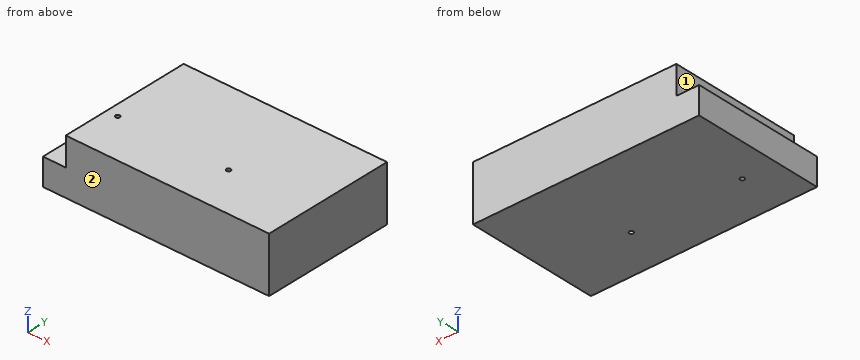
from build123d import *

# Parameters (mm, degrees)
SKETCH_1_W          = 159
SKETCH_1_H          = 93
EXTRUDE_1_DEPTH     = 39
SKETCH_2_R          = 1.5
CUT_EXTRUDE_1_DEPTH = 39
SKETCH_3_W          = 16
SKETCH_3_H          = 93
CUT_EXTRUDE_2_DEPTH = 20


with BuildPart() as part:
    # Эскиз1 → Бобышка-Вытянуть1 (new body)
    with BuildSketch(Plane.XY):
        Rectangle(SKETCH_1_W, SKETCH_1_H)
    extrude(amount=EXTRUDE_1_DEPTH)

    # Эскиз2 → Вырез-Вытянуть1 (cut)
    with BuildSketch(Plane(origin=(0, 0, 0), x_dir=(-1, 0, 0), z_dir=(0, 0, -1))):
        with Locations((-22.5, -14.5)):
            Circle(SKETCH_2_R)
        with Locations((55.5, -14.5)):
            Circle(SKETCH_2_R)
    extrude(amount=-CUT_EXTRUDE_1_DEPTH, mode=Mode.SUBTRACT)

    # Эскиз3 → Вырез-Вытянуть2 (cut)
    with BuildSketch(Plane.XY.offset(39)):
        with Locations((-71.5, 0)):
            Rectangle(SKETCH_3_W, SKETCH_3_H)
    extrude(amount=-CUT_EXTRUDE_2_DEPTH, mode=Mode.SUBTRACT)


solid = part.part
Geometry: final body of the model. Coordinates: model frame, mm. Face numbers are marked on the shaded views. A direction names the side the tool comes from. Give positions to 0.01 mm unless a question says otherwise; leave off trailing zeros. Write each loop counter-clockwise with the first axis right and the second up, starting at its lowest first coordinate (ties: lowest second). Pieces come first, ordered by that corner, then holes. Notation, with made-up numbers: (56.5, 27) -> (67.5, 27) arc R22 cw to (67.5, 35) -> close; hole circle Ø8 at (-15, 83). An arc over 180 degrees is marked (long way). Answer as a JSON object with one key per item and string values.
1. Ray query, probe 1 along X at (y, z) = (-14, 10); probe 2 along Y at (x, z) = (22.5, 31); probe 3 along X at (y, z) = (-9, 26.5). Return the intervals inside material, ascending. Write a range as from..to.
Ans:
{"probe 1": "x = -79.5..-56.91, -54.09..21.09, 23.91..79.5", "probe 2": "y = -46.5..-16, -13..46.5", "probe 3": "x = -63.5..79.5"}
2. Contact query for flat-ended pins moving along their axis: pin 1 (8 mm diameter, centred on x = -73.5, y = 13.5, fed in from +Z); pin 2 (1.5 mm diameter, centred on x = -56, y = -23, fed in from -Z); pin 3 (16 mm diameter, centred on y = 10.5, z = 29.5, fed in from -X). Output: stop coordinate, or through.
Ans:
{"pin 1": "stops at z = 19", "pin 2": "stops at z = 0", "pin 3": "stops at x = -63.5"}
3. Cut plane A-A on z = 36. Output: boundary loops of the cut face in (x, y), and give its area (3 significant figures).
Ans:
{"outline": "(-63.5, -46.5) -> (79.5, -46.5) -> (79.5, 46.5) -> (-63.5, 46.5) -> close; hole circle Ø3 at (-55.5, -14.5); hole circle Ø3 at (22.5, -14.5)", "area": "13,300 mm^2"}
4. Cut plane B-B on y = -20.5. Output: boundary loops of the cut face in (x, z), and give its area (3 significant figures).
Ans:
{"outline": "(-79.5, 0) -> (79.5, 0) -> (79.5, 39) -> (-63.5, 39) -> (-63.5, 19) -> (-79.5, 19) -> close", "area": "5,880 mm^2"}
5. Access query for the marked faces 1 and 2. Directions: +Z, -Z, +X, -X, +Y, -Y. A direction counts if a zero-diameter tool reaches every point of the face in a straight line with its end or side. Return the directions, or none.
Ans:
{"face 1": "+Z, -X, +Y, -Y", "face 2": "+Z, -Z, +X, -X, -Y"}
